Can you work these out from the model? Positions are in its coordinate system, mm. Face numbers are marked on the shaded views. A direction names the side the tool comes from. Coordinates: 2 decimals unless noted, no trailing zeros. Order: outer loops, then holes, each group sorted by start corner. A loop starts at its lowest first (then second) coordinate and runs counter-clockwise, first axis right, second up. Notation, with made-up numbers: (-11, 77.5) - (34, 77.5) arc R18 cw to (34, 92.5) - close; hole circle Ø3 at (-27.5, -1). An arc over 180 degrees is marked (long way). Return JSON: item names as keys, results as strings. Group by question number.
1) Imagine slicing it at B-B (z = -11.25). Write out the boundary of the cut face in (x, y), and give its area (3 significant figures).
2) If we mould it in two halves opening along X, with no side actions, what happens to the marked faces 3, 4 and 5? For each: pulls with the +X half, pulls with the -X half, needs draft (parallel to the pull), parting line crosses it, or undercut.
3) Which directions (+Z, -Z, +X, -X, +Y, -Y) give clear straight access to the entire face, cutting with the end or side of a thin tool? Please do the marked faces 1 and 2.
4) For pin 1 Ø1 at (y, z) = (1.5, -10.5) entering from +X; pin 2 Ø2 at (y, z) = (0.5, -9.5) entering from -X, each with a flat end and sliding along its axis, tell me the tip position at first contact or that it passes through.
5) Imagine slicing it at A-A (x = 0). Write out the boundary of the cut face in (y, z).
6) If I drill on line 1 along Z through (x, y) = (-0.3, -0.35); line 2 along Z through (x, y) = (1.7, 0.1); line 3 along X through (y, z) = (0.95, -8.25), over which ranges is the centre line in solid material (lowest first)?
Autodesk Inventor part; units mm, degrees
ref_plane "YZ Plane" through (0, 0, 0) normal (1, 0, 0) x (0, 1, 0)
ref_plane "XZ Plane" through (0, 0, 0) normal (0, 1, 0) x (-1, 0, 0)
ref_plane "XY Plane" through (0, 0, 0) normal (0, 0, 1) x (1, 0, 0)
sketch "Sketch1" plane through (0, 0, 0) normal (1, 0, 0) x (0, 1, 0)
  line L0 (0, 0) -> (0, -16)
  line L1 (0, -16) -> (3, -16)
  line L2 (3, -16) -> (1.5, -14.5)
  line L3 (1.5, -14.5) -> (1.5, 0)
  line L4 (1.5, 0) -> (0, 0)
  dimension "d0" = 6
  dimension "d1" = 16
  dimension "d2" = 45
  dimension "d3" = 3
revolve "Revolution1" add sketch "Sketch1" angle 360 about axis through (0, 0, 0) along (0, 0, -1)
chamfer "Chamfer1" distance 0.2 angle 45 1 edges at (0, -1.5, 0)
thread "Thread1"
sketch "Sketch2" plane through (0, 0, -16) normal (0, 0, -1) x (-1, 0, 0)
  circle A0 centre (0, 0) radius 1.3
  line L0 (1.1547, 0) -> (0.5774, -1)
  line L1 (0.5774, -1) -> (-0.5774, -1)
  line L2 (-0.5774, -1) -> (-1.1547, 0)
  line L3 (-1.1547, 0) -> (-0.5774, 1)
  line L4 (-0.5774, 1) -> (0.5774, 1)
  line L5 (0.5774, 1) -> (1.1547, 0)
  dimension "d10" = 2
extrude "Extrusion1" cut sketch "Sketch2" against normal blind 1.2 contours L0 L1 L2 L3 L4 L5
properties part number "M3 x 16mm FHCS"
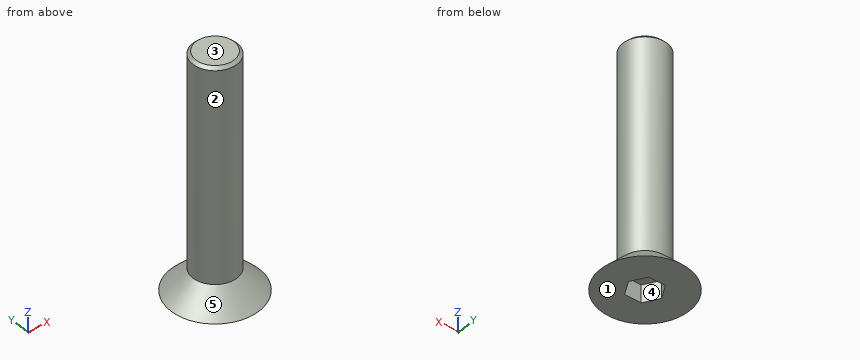
Calculated:
{
 "1": {"outline": "circle Ø3 at (0, 0)", "area": "7.07 mm2"},
 "2": {"face 3": "needs draft", "face 4": "undercut", "face 5": "parting line crosses it"},
 "3": {"face 1": "-Z, +X, -X, +Y, -Y", "face 2": "+Z"},
 "4": {"pin 1": "x = 1.12", "pin 2": "x = -1.5"},
 "5": {"outline": "(-3, -16) - (-1, -16) - (-1, -14.8) - (1, -14.8) - (1, -16) - (3, -16) - (1.5, -14.5) - (1.5, -0.2) - (1.3, 0) - (-1.3, 0) - (-1.5, -0.2) - (-1.5, -14.5) - close"},
 "6": {"line 1": "-14.8 to 0", "line 2": "-16 to -14.7", "line 3": "-1.16 to 1.16"}
}
